```python
from build123d import *

# Parameters (mm, degrees)
BOSS_EXTRUDE1_DEPTH = 20
BOSS_EXTRUDE2_START = -1
BOSS_EXTRUDE2_DEPTH = 1
SKETCH3_R           = 1.5
CUT_EXTRUDE1_DEPTH  = 44.239768732
SKETCH4_R           = 2.0828
CUT_EXTRUDE2_DEPTH  = 41.983869998


with BuildPart() as part:
    # Sketch1 → Boss-Extrude1 (new body)
    with BuildSketch(Plane.XY):
        with BuildLine():
            Line((-16.5, 0), (-31.74, 0))
            Line((-31.74, 0), (-31.74, 5))
            Line((-31.74, 5), (-20.910523666, 5))
            ThreePointArc((-20.910523666, 5), (0, 21.5), (20.910523666, 5))
            Line((20.910523666, 5), (31.74, 5))
            Line((31.74, 5), (31.74, 0))
            Line((31.74, 0), (16.5, 0))
            ThreePointArc((16.5, 0), (0, 16.5), (-16.5, 0))
        make_face()
    extrude(amount=BOSS_EXTRUDE1_DEPTH)

    # Sketch2 → Boss-Extrude2 (add)
    with BuildSketch(Plane.XY.offset(20).offset(BOSS_EXTRUDE2_START)):
        with BuildLine():
            Line((5, 0), (16.5, 0))
            ThreePointArc((16.5, 0), (0, 16.5), (-16.5, 0))
            Line((-16.5, 0), (-5, 0))
            Line((-5, 0), (-5, 6))
            ThreePointArc((-5, 6), (0, 11), (5, 6))
            Line((5, 6), (5, 0))
        make_face()
    extrude(amount=BOSS_EXTRUDE2_DEPTH)

    # Sketch3 → Cut-Extrude1 (cut, through all)
    with BuildSketch(Plane.XY.offset(20)):
        with Locations((-11.691342951, 6.75)):
            Circle(SKETCH3_R)
        with Locations((11.691342951, 6.75)):
            Circle(SKETCH3_R)
    extrude(amount=-CUT_EXTRUDE1_DEPTH, mode=Mode.SUBTRACT)

    # Sketch4 → Cut-Extrude2 (cut, through all)
    with BuildSketch(Plane(origin=(0, 5, 0), x_dir=(1, 0, 0), z_dir=(0, 1, 0))):
        with Locations(Location((26.325261833, -10, 0), (0, 0, 180))):
            Circle(SKETCH4_R)
        with Locations((-26.325261833, -10)):
            Circle(SKETCH4_R)
    extrude(amount=-CUT_EXTRUDE2_DEPTH, mode=Mode.SUBTRACT)


solid = part.part
```
CAD build for the part. Positions are in the model's coordinates, mm. A direction names the side the tool comes from. Give positions to 0.01 mm unless a question says otherwise; leave off trailing zeros. Write each loop counter-clockwise with the first axis right and the second up, starting at its lowest first coordinate (ties: lowest second). Pieces come first, ordered by that corner, then holes. Notation, with made-up numbers: M 59.5,30.5 L 115.5,30.5 A28 ccw 115.5,61.5 Z; hole C 51,21.5 d9. An arc over 180 degrees is marked long. Return JSON: item names as keys, results as strings. Group by question number.
(1) Mould opens along Y. For faces 4 (the face through (-13.19, 6.82, 19.51)), 5 (the face through (-26.4, 5, 7.6)), 6 (the face through (31.74, 3, 10)), 7 (the face through (12.384, 5.419, 19.507)) say: pulls with the +Y half, pulls with the -Y half, needs draft (parallel to the pull), parting line crosses it, or undercut.
(2) 3-axis set-ups, long thin cutter, end or side, ignore diameter. For faces 1 (the face through (26.2, 5, 7.6)), 2 (the face through (0, 12, 19)), 3 (the face through (-0.402, 21.496, 9.86)): which of +Z, -Z, +X, -X, +Y, -Y reach the whole face in a straight line?
(3) Band-saw the part on B-B (z = 15.5). Give the cut face in (x, y).
(4) Drill centre lines: L1, parallel to Z at x = -4, y = 9.75; L2, parallel to Y at x = -0.5, z = 3.75; L3, parallel to X at y = 6.75, z = 9.25. Where is each one in solid material? Low to high. Write a range as [from, to].
(5) Band-saw the part on D-D (z = 10). Give the cut face in (x, y), and give its area (3 significant figures).
(6) Band-saw the part on C-C (x = 27). Give the cut face in (y, z).
(7) Band-saw the part on A-A (y = 1.5). Give the cut face in (x, z), and give its area (3 significant figures).
(8) Flat gauge pins, fed straight in: pin 1 Ø5.5 at (x, z) = (26.5, 6.5) entering from +Y; pin 2 Ø4 at (x, y) = (11.69, 6.75) entering from -Z; pin 3 Ø2.5 at (x, y) = (-11.69, 6.75) entering from +Z; pin 4 Ø5 at (y, z) = (13, 6) entering from -X. Where does each tip first touch, or does it go through?
Entries:
{
 "1": {"face 4": "undercut", "face 5": "pulls with the +Y half", "face 6": "needs draft", "face 7": "undercut"},
 "2": {"face 1": "+Z, -Z, +X, +Y", "face 2": "-Z, -Y", "face 3": "+Z, -Z, +Y"},
 "3": {"outline": "M -31.74,0 L -16.5,0 A16.5 cw 16.5,0 L 31.74,0 L 31.74,5 L 20.91,5 A21.5 ccw -20.91,5 L -31.74,5 Z"},
 "4": {"L1": "z = [19, 20]", "L2": "y = [16.49, 21.49]", "L3": "x = [-20.41, -15.06], [15.06, 20.41]"},
 "5": {"outline": "M -31.74,0 L -28.41,0 L -28.41,5 L -31.74,5 Z; M -24.24,0 L -16.5,0 A16.5 cw 16.5,0 L 24.24,0 L 24.24,5 L 20.91,5 A21.5 ccw -20.91,5 L -24.24,5 Z; M 28.41,0 L 31.74,0 L 31.74,5 L 28.41,5 Z", "area": "361 mm^2"},
 "6": {"outline": "M 0,0 L 5,0 L 5,8.03 L 0,8.03 Z; M 0,11.97 L 5,11.97 L 5,20 L 0,20 Z"},
 "7": {"outline": "M -31.74,0 L -16.43,0 L -16.43,19 L -5,19 L -5,20 L -31.74,20 Z; M 5,19 L 16.43,19 L 16.43,0 L 31.74,0 L 31.74,20 L 5,20 Z; hole C -26.33,10 d4.17; hole C 26.33,10 d4.17", "area": "608 mm^2"},
 "8": {"pin 1": "stops at y = 5", "pin 2": "stops at z = 19", "pin 3": "passes through", "pin 4": "stops at x = -18.76"}
}
